CAD build for the part. Positions are in the model's coordinates, mm. Face numbers are marked on the shaded views. A direction names the side the tool comes from. Coordinates: 2 decimals unless noted, no trailing zeros. Loops run counter-clockwise (first coordinate to the right, second up) from the corner with the lowest first, then second, coordinate; pieces in that order, holes last.
1) Pin check, flat tips, straight feed: pin 1 Ø4 at (x, y) = (-5, 10) entering from -Z; pin 2 Ø2 at (x, y) = (-1, 31.5) entering from -Z; pin 3 Ø5 at (x, y) = (2, 31) entering from +Z; pin 4 Ø8 at (x, z) = (0.5, 1.5) entering from +Y. Stop position of each tip, or through.
2) Saw through at C-C, the plane y = 15. Write the cut outline in (x, z), and give its area (3 significant figures).
3) Saw through at A-A, the plane z = 0. Write the cut outline in (x, y).
4) Wall check: line 1 along X through (y, z) = (42.55, 0); line 2 along Y through (x, z) = (1.5, 5.5); line 3 along Y through (x, z) = (0, -0.5). Give the ranges that are in metal, low to high.
5) Two-plate mould, pull along X, no slides. Class the marked faces 1, 2 and 3: +X half, -X half, draft (parallel to the pull), parting line (faces both ways), or undercut.
6) Saw through at D-D, the plane z = -4.25. Write the cut outline in (x, y), and give its area (3 significant figures).
7) Saw through at B-B, the plane x = 0. Write the cut outline in (y, z).
8) Which spindle directions (+Z, -Z, +X, -X, +Y, -Y) get a long thin tool onto all of the face, cutting with end or side? Do the marked faces 4 and 5. Say none if no direction does.
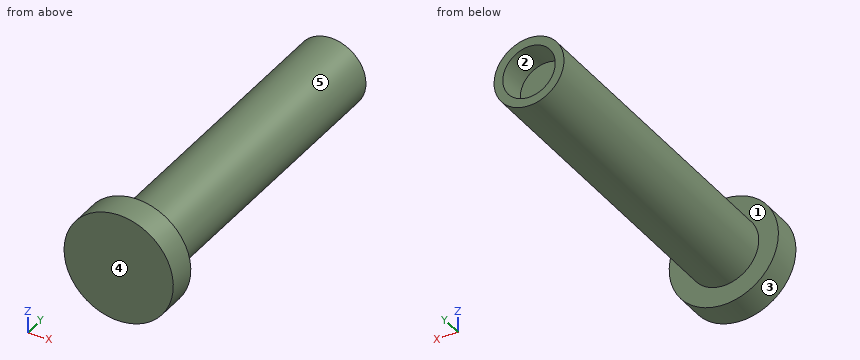
```python
from build123d import *

# Parameters (mm, degrees)
SKETCH1_R           = 4.8
BOSS_EXTRUDE1_DEPTH = 44.45
SKETCH1_4_R         = 7.5
SKETCH1_4_R_2       = 4.8
BOSS_EXTRUDE2_DEPTH = 4
SKETCH2_R           = 3.6
CUT_EXTRUDE1_DEPTH  = 4


with BuildPart() as part:
    # Sketch1 → Boss-Extrude1 (new body)
    with BuildSketch(Plane(origin=(0, 0, 0), x_dir=(1, 0, 0), z_dir=(0, 1, 0))):
        with Locations(Location((0, 0, 0), (0, 0, 270))):
            Circle(SKETCH1_R)
    extrude(amount=BOSS_EXTRUDE1_DEPTH)

    # Sketch1_4 → Boss-Extrude2 (add)
    with BuildSketch(Plane(origin=(0, 0, 0), x_dir=(1, 0, 0), z_dir=(0, 1, 0))):
        with Locations(Location((0, 0, 0), (0, 0, 270))):
            Circle(SKETCH1_4_R)
        with Locations(Location((0, 0, 0), (0, 0, 270))):
            Circle(SKETCH1_4_R_2, mode=Mode.SUBTRACT)
        with Locations(Location((0, 0, 0), (0, 0, 270))):
            Circle(SKETCH1_4_R_2)
    extrude(amount=-BOSS_EXTRUDE2_DEPTH)

    # Sketch2 → Cut-Extrude1 (cut)
    with BuildSketch(Plane(origin=(0, 44.45, 0), x_dir=(1, 0, 0), z_dir=(0, 1, 0))):
        with Locations(Location((0, 0, 0), (0, 0, 270))):
            Circle(SKETCH2_R)
    extrude(amount=-CUT_EXTRUDE1_DEPTH, mode=Mode.SUBTRACT)


solid = part.part
```
Data:
1. pin 1: stops at z = -3.75
1. pin 2: stops at z = -4.8
1. pin 3: stops at z = 4.8
1. pin 4: stops at y = 44.45
2. outline: circle Ø9.6 at (0, 0)
2. area: 72.4 mm2
3. outline: (-7.5, -4) - (7.5, -4) - (7.5, 0) - (4.8, 0) - (4.8, 44.45) - (3.6, 44.45) - (3.6, 40.45) - (-3.6, 40.45) - (-3.6, 44.45) - (-4.8, 44.45) - (-4.8, 0) - (-7.5, 0) - close
4. line 1: x = -4.8 to -3.6, 3.6 to 4.8
4. line 2: y = -4 to 0
4. line 3: y = -4 to 40.45
5. face 1: draft
5. face 2: undercut
5. face 3: parting line
6. outline: (-6.18, -4) - (6.18, -4) - (6.18, 0) - (2.23, 0) - (2.23, 44.45) - (-2.23, 44.45) - (-2.23, 0) - (-6.18, 0) - close
6. area: 248 mm2
7. outline: (-4, -7.5) - (0, -7.5) - (0, -4.8) - (44.45, -4.8) - (44.45, -3.6) - (40.45, -3.6) - (40.45, 3.6) - (44.45, 3.6) - (44.45, 4.8) - (0, 4.8) - (0, 7.5) - (-4, 7.5) - close
8. face 4: +Z, -Z, +X, -X, -Y
8. face 5: +Y
